Drawing for the job (mm, zero at the part's lowest x, y, z). A direction names the side the tool comes from. Give positions to 0.01 mm unless a question says otherwise; leave off trailing zeros. Order: outer loops, then holes, each group sorted by start corner. A loop starts at its lowest first (then second) coordinate and runs counter-clockwise, first axis right, second up. Notation, with made-up numbers: (66, 27.5) - (88, 27.5) arc R24 cw to (88, 52.5) - close; hole circle Ø3 at (69.25, -31). An arc over 180 degrees is marked (long way). Use a Markdown table: item, result.
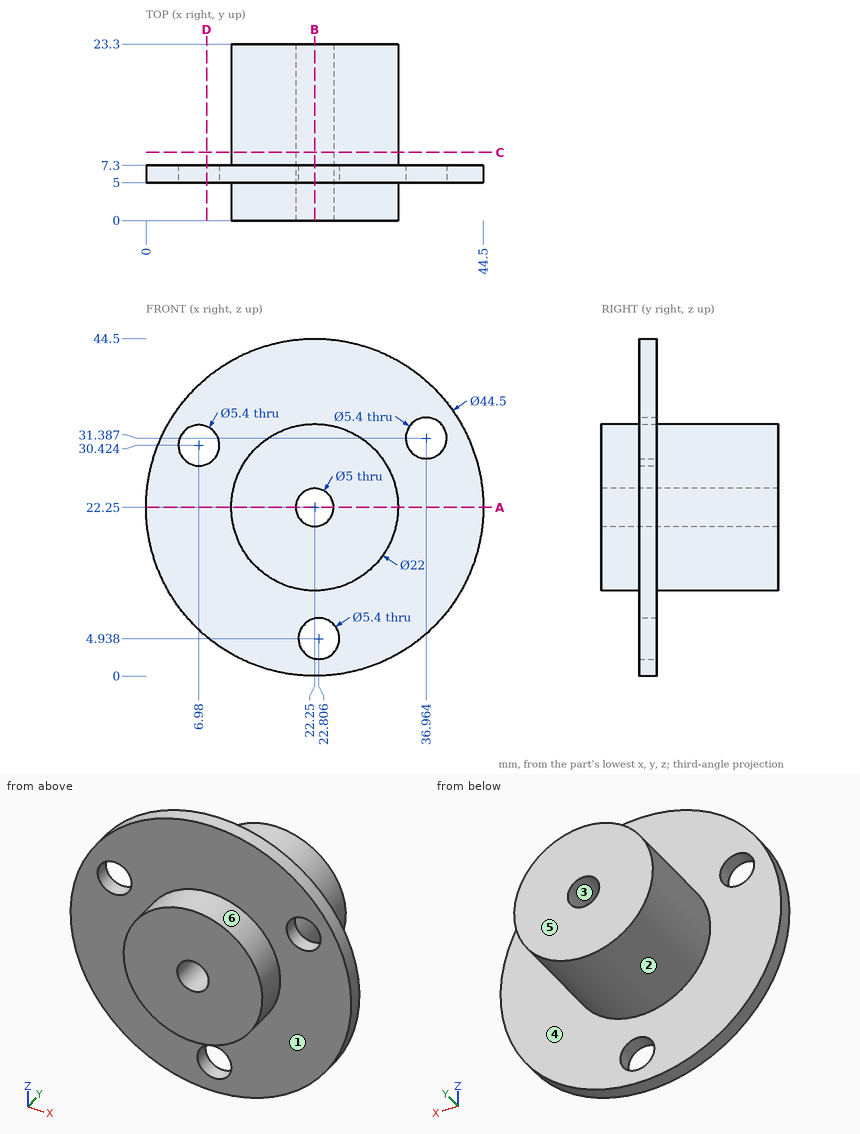
1) Two-plate mould, pull along X, no slides. Class the marked faces 1, 2 and 3: +X half, -X half, draft (parallel to the pull), parting line (faces both ways), or undercut.
Computed:
| item | result |
|---|---|
| face 1 | draft |
| face 2 | parting line |
| face 3 | undercut |
2) Wall check: line 1 (Z direction, x = 22.5, y = 2.5); line 2 (X direction, y = 18.25, z = 22.25); line 3 (Y direction, x = 4, z = 18.5). Give the ranges that are in metal, low to high. Write a range as from..to.
Computed:
| item | result |
|---|---|
| line 1 | z = 11.25..19.76, 24.74..33.25 |
| line 2 | x = 11.25..19.75, 24.75..33.25 |
| line 3 | y = 5..7.3 |
3) Slice it at C-C (y = 9). Write the cut outline in (x, z).
Computed:
| item | result |
|---|---|
| outline | circle Ø22 at (22.25, 22.25); hole circle Ø5 at (22.25, 22.25) |
4) Slice it at A-A (z = 22.25). Write the cut outline in (x, y), and give its area (3 significant figures).
Computed:
| item | result |
|---|---|
| outline | (0, 5) - (11.25, 5) - (11.25, 0) - (19.75, 0) - (19.75, 23.3) - (11.25, 23.3) - (11.25, 7.3) - (0, 7.3) - close; (24.75, 0) - (33.25, 0) - (33.25, 5) - (44.5, 5) - (44.5, 7.3) - (33.25, 7.3) - (33.25, 23.3) - (24.75, 23.3) - close |
| area | 448 mm² |
5) Slice it at D-D (x = 8). Write the cut outline in (y, z) (1 decimal).
Computed:
| item | result |
|---|---|
| outline | (5, 5.2) - (7.3, 5.2) - (7.3, 27.9) - (5, 27.9) - close; (5, 32.9) - (7.3, 32.9) - (7.3, 39.3) - (5, 39.3) - close |
6) Slice it at B-B (x = 22.25). Write the cut outline in (y, z).
Computed:
| item | result |
|---|---|
| outline | (0, 11.25) - (5, 11.25) - (5, 7.58) - (7.3, 7.58) - (7.3, 11.25) - (23.3, 11.25) - (23.3, 19.75) - (0, 19.75) - close; (0, 24.75) - (23.3, 24.75) - (23.3, 33.25) - (7.3, 33.25) - (7.3, 44.5) - (5, 44.5) - (5, 33.25) - (0, 33.25) - close; (5, 0) - (7.3, 0) - (7.3, 2.3) - (5, 2.3) - close |
7) Pin check, flat tips, straight feed: P1, Ø2, axis at x = 14, y = 6, coming from the +Z side (1 decimal); P2, Ø22, axis at x = 14, z = 13.5, coming from the -Y side; P3, Ø1, axis at x = 26, y = 3, coming from the +Z side; P4, Ø1, axis at x = 31, y = 18, coming from the +Z side (1 decimal). Stop position of each tip, or through.
Computed:
| item | result |
|---|---|
| P1 | stops at z = 43.3 |
| P2 | stops at y = 0 |
| P3 | stops at z = 32.76 |
| P4 | stops at z = 29.5 |
8) Tool access for the marked faces 4, 5 and 6: list every direction of +Z, -Z, +X, -X, +Y, -Y with a clear straight run to the whole face (end or side of a thin tool).
Computed:
| item | result |
|---|---|
| face 4 | +Y |
| face 5 | +Z, -Z, +X, -X, +Y |
| face 6 | -Y |
